```python
from build123d import *

# Parameters (mm, degrees)
BASE_FLANGE1_DEPTH       = 2.5
FILLET1_RADIUS           = 2.5
FILLET1_LENGTH           = 0.75
FILLET2_RADIUS           = 2.5
FILLET2_LENGTH           = 0.75
M2_CLEARANCE_HOLE1_D     = 2.4
M2_CLEARANCE_HOLE1_DEPTH = 6
M2_CLEARANCE_HOLE1_TIP   = 0.721032743
M2_CLEARANCE_HOLE2_D     = 2.4
M2_CLEARANCE_HOLE2_DEPTH = 6
M2_CLEARANCE_HOLE2_TIP   = 0.721032743


# Sheet-metal steps are written as plain solids
with BuildPart() as part:
    # Sketch1 → Base-Flange1 (new, symmetric)
    with BuildSketch(Plane(origin=(0, 0, 0), x_dir=(0, 0, -1), z_dir=(1, 0, 0))):
        with BuildLine():
            Line((0, 19.75), (0, 1))
            ThreePointArc((0, 1), (0.292893219, 0.292893219), (1, 0))
            Line((1, 0), (7.5, 0))
            Line((7.5, 0), (7.5, 0.75))
            Line((7.5, 0.75), (1, 0.75))
            ThreePointArc((1, 0.75), (0.823223305, 0.823223305), (0.75, 1))
            Line((0.75, 1), (0.75, 19.75))
            Line((0.75, 19.75), (0, 19.75))
        make_face()
    extrude(amount=BASE_FLANGE1_DEPTH, both=True)

    # Fillet1: full round fillet: the end face becomes a half cylinder, R = half its width
    fillet1_face = Plane((0, 0.375, -7.5), x_dir=(0, -1, 0), z_dir=(0, 0, -1))  # on the end face: x along it, z out of the body
    fillet1_slab = fillet1_face.offset(-FILLET1_RADIUS / 2) * Box(FILLET1_LENGTH, 2 * FILLET1_RADIUS, FILLET1_RADIUS, mode=Mode.PRIVATE)  # the body's end, R deep
    fillet1_round = Plane((0, 0.375, -5), x_dir=(0, 0, -1), z_dir=(0, -1, 0)) * Cylinder(FILLET1_RADIUS, FILLET1_LENGTH, mode=Mode.PRIVATE)  # its axis R under the face
    add(fillet1_slab - fillet1_round, mode=Mode.SUBTRACT)

    # Fillet2: full round fillet: the end face becomes a half cylinder, R = half its width
    fillet2_face = Plane((0, 19.75, -0.375), x_dir=(0, 0, -1), z_dir=(0, 1, 0))  # on the end face: x along it, z out of the body
    fillet2_slab = fillet2_face.offset(-FILLET2_RADIUS / 2) * Box(FILLET2_LENGTH, 2 * FILLET2_RADIUS, FILLET2_RADIUS, mode=Mode.PRIVATE)  # the body's end, R deep
    fillet2_round = Plane((0, 17.25, -0.375), x_dir=(0, 1, 0), z_dir=(0, 0, -1)) * Cylinder(FILLET2_RADIUS, FILLET2_LENGTH, mode=Mode.PRIVATE)  # its axis R under the face
    add(fillet2_slab - fillet2_round, mode=Mode.SUBTRACT)

    # M2 Clearance Hole1
    with Locations(Plane.XY):
        with Locations((0, 17.25)):
            Hole(M2_CLEARANCE_HOLE1_D / 2, depth=M2_CLEARANCE_HOLE1_DEPTH)
            with Locations((0, 0, -(M2_CLEARANCE_HOLE1_DEPTH + M2_CLEARANCE_HOLE1_TIP / 2))):  # 118° drill point
                Cone(0, M2_CLEARANCE_HOLE1_D / 2, M2_CLEARANCE_HOLE1_TIP, mode=Mode.SUBTRACT)

    # M2 Clearance Hole2
    with Locations(Plane(origin=(0, 0.75, 0), x_dir=(1, 0, 0), z_dir=(0, 1, 0))):
        with Locations((0, 5)):
            Hole(M2_CLEARANCE_HOLE2_D / 2, depth=M2_CLEARANCE_HOLE2_DEPTH)
            with Locations((0, 0, -(M2_CLEARANCE_HOLE2_DEPTH + M2_CLEARANCE_HOLE2_TIP / 2))):  # 118° drill point
                Cone(0, M2_CLEARANCE_HOLE2_D / 2, M2_CLEARANCE_HOLE2_TIP, mode=Mode.SUBTRACT)


solid = part.part
```
Verification items for the finished model (mm, model axes). A direction names the side the tool comes from. Round coordinates to 2 decimals unless told otherwise and drop trailing zeros. Write each loop counter-clockwise with the first axis right and the second up, starting at its lowest first coordinate (ties: lowest second). Pieces come first, ordered by that corner, then holes.
1. Draft check along Z on faces 1 (the flat face through (-2.5, 7.4, -0.6)), 2 (the cylindrical face through (-0.65, 0.37, -6.01)), 3 (the cylindrical face through (-0.1, 0.4, -7.5)). Enter one of: +Z half, -Z half, draft (parallel to the pull), parting line (faces both ways), or undercut.
2. Section check C-C on x = 1.5. Enter the section's corners in (y, z).
3. Gauge pin test, flat end, axial feed: P1, Ø1.5, axis at x = -1, z = -2, coming from the +Y side. Record the tip position at first contact, or that the pin passes through.
4. Section check A-A on x = 0. Enter the section's corners in (y, z).
5. Section check B-B on z = -4.25. Enter the section's corners in (x, y), plus the area to 3 significant figures.
6. Section check D-D on y = 1.25. Enter the section's corners in (x, z), plus the area to 3 significant figures.
7. Access from +Z, -Z, +X, -X, +Y, -Y to the whole of each face (thin tool, end or side, straight path). Record for faces 4 (the cylindrical face through (-0.05, 19.75, -0.38)), 5 (the flat face through (0, 0.75, -3.6)).
8. Scan lines: L1, parallel to X at y = 0.2, z = -5; L2, parallel to Z at x = -1.7, y = 5.75; L3, parallel to Z at x = 0, y = 0.5. Record each from-to range of solid material in increasing order.
Answer:
1. face 1: draft
1. face 2: undercut
1. face 3: -Z half
2. outline: (0, -7) - (0.75, -7) - (0.75, -1) arc R0.25 cw to (1, -0.75) - (19.25, -0.75) - (19.25, 0) - (1, 0) arc R1 ccw to (0, -1) - close
3. P1: stops at y = 0.75
4. outline: (0, -7.5) - (0.75, -7.5) - (0.75, -6.2) - (0, -6.2) - close; (0, -3.8) - (0.75, -3.8) - (0.75, -1) arc R0.25 cw to (1, -0.75) - (16.05, -0.75) - (16.05, 0) - (1, 0) arc R1 ccw to (0, -1) - close; (18.45, -0.75) - (19.75, -0.75) - (19.75, 0) - (18.45, 0) - close
5. outline: (-2.5, 0) - (-0.94, 0) - (-0.94, 0.75) - (-2.5, 0.75) - close; (0.94, 0) - (2.5, 0) - (2.5, 0.75) - (0.94, 0.75) - close
5. area: 2.34 mm2
6. outline: (-2.5, -0.75) - (2.5, -0.75) - (2.5, 0) - (-2.5, 0) - close
6. area: 3.75 mm2
7. face 4: +Z, -Z, +Y
7. face 5: -Z, +X, -X, +Y
8. L1: x = -2.5 to -1.2, 1.2 to 2.5
8. L2: z = -0.75 to 0
8. L3: z = -7.5 to -6.2, -3.8 to -0.13
